```python
from build123d import *

# Parameters (mm, degrees)
BOSS_EXTRUDE1_DEPTH = 35
SKETCH3_W           = 28
SKETCH3_H           = 14
CUT_EXTRUDE1_DEPTH  = 4
FILLET1_R           = 1
SKETCH4_R           = 2
CUT_EXTRUDE2_DEPTH  = 63.072538211


with BuildPart() as part:
    # Sketch2 → Boss-Extrude1 (new body)
    with BuildSketch(Plane.XY):
        Polygon((0, 0), (0, 2), (10, 2), (10, 18), (38, 18), (38, 2), (48, 2), (48, 0), (36, 0), (36, 16), (12, 16), (12, 0), align=None)
    extrude(amount=BOSS_EXTRUDE1_DEPTH)

    # Sketch3 → Cut-Extrude1 (cut)
    with BuildSketch(Plane(origin=(0, 18, 0), x_dir=(1, 0, 0), z_dir=(0, 1, 0))):
        with Locations((24, -28)):
            Rectangle(SKETCH3_W, SKETCH3_H)
    extrude(amount=-CUT_EXTRUDE1_DEPTH, mode=Mode.SUBTRACT)

    # Fillet1
    fillet1_edges = [part.edges().sort_by_distance(p)[0] for p in [
        (0, 2, 17.5),
        (48, 2, 17.5),
        (10, 18, 10.5),
        (38, 18, 10.5),
    ]]
    fillet(fillet1_edges, radius=FILLET1_R)

    # Sketch4 → Cut-Extrude2 (cut, through all)
    with BuildSketch(Plane(origin=(0, 18, 0), x_dir=(1, 0, 0), z_dir=(0, 1, 0))):
        with Locations(Location((24, -8, 0), (0, 0, 270))):
            Circle(SKETCH4_R)
        with Locations(Location((24, -16, 0), (0, 0, 270))):
            Circle(SKETCH4_R)
        with Locations(Location((42.5, -5, 0), (0, 0, 270))):
            Circle(SKETCH4_R)
        with Locations(Location((42.5, -30, 0), (0, 0, 270))):
            Circle(SKETCH4_R)
        with Locations(Location((4.5, -5, 0), (0, 0, 270))):
            Circle(SKETCH4_R)
        with Locations(Location((4.5, -30, 0), (0, 0, 270))):
            Circle(SKETCH4_R)
    extrude(amount=-CUT_EXTRUDE2_DEPTH, mode=Mode.SUBTRACT)


solid = part.part
```
CAD build for the part. Positions are in the model's coordinates, mm. A direction names the side the tool comes from. Coordinates: 2 decimals unless noted, no trailing zeros. Write each loop counter-clockwise with the first axis right and the second up, starting at its lowest first coordinate (ties: lowest second). Pieces come first, ordered by that corner, then holes. Notation, with made-up numbers: (22, 59) -> (39, 59) arc R28 ccw to (39, 77) -> close; hole circle Ø10 at (34, 77.25). An arc over 180 degrees is marked (long way). Use CSV: the item, a comma, the result in double quotes. Start each with the question number.
Item 1: Wall check: probe 1 along X at (y, z) = (0.6, 30); probe 2 along X at (y, z) = (15.25, 3); probe 3 along X at (y, z) = (16.7, 8). Give the ranges that are in metal, low to high.
Item 2: Band-saw the part on D-D, the plane y = 7. Write the cut outline in (x, z).
Item 3: Tool access for faces 1 (the flat face through (48, 0.5, 17.3)), 2 (the flat face through (12, 8, 17)), 3 (the flat face through (38, 10, 17)), 4 (the cylindrical face through (4.588, 1.014, 3.002)), 5 (the flat face through (5, 2, 17)): list every direction of +Z, -Z, +X, -X, +Y, -Y with a clear straight run to the whole face (end or side of a thin tool).
Item 4: Drop flat-ended pins along their axis: P1, Ø1.6, axis at x = 37, z = 27.5, coming from the +Y side; P2, Ø3, axis at x = 26, y = 15, coming from the +Z side; P3, Ø5, axis at y = 4, z = 15.5, coming from the -X side. Give the stop position or say it passes through.
Item 5: Band-saw the part on B-B, the plane y = 14.5. Write the cut outline in (x, z).
Item 6: Two-plate mould, pull along X, no slides. Class faces 6 (the flat face through (0, 0.5, 17.3)), 7 (the flat face through (37.6, 5, 35)), 8 (the flat face through (24.2, 16, 10.4)): +X half, -X half, draft (parallel to the pull), parting line (faces both ways), or undercut.
Item 7: Band-saw the part on C-C, the plane z = 30. Write the cut outline in (x, y), plus the area to 3 significant figures.
Item 8: Band-saw the part on A-A, the plane z = 8. Write the cut outline in (x, y), plus the area to 3 significant figures.
Response values:
1,probe 1,"x = 0 to 2.5, 6.5 to 12, 36 to 40.5, 44.5 to 48"
1,probe 2,"x = 10 to 12, 36 to 38"
1,probe 3,"x = 10 to 22, 26 to 38"
2,outline,"(10, 0) -> (12, 0) -> (12, 35) -> (10, 35) -> close; (36, 0) -> (38, 0) -> (38, 35) -> (36, 35) -> close"
3,face 1,"+Z, -Z, +X, +Y, -Y"
3,face 2,"+Z, -Z, -Y"
3,face 3,"+Z, -Z, +X, +Y"
3,face 4,"+Y, -Y"
3,face 5,"+Z, -Z, -X, +Y"
4,P1,"stops at y = 14"
4,P2,"stops at z = 21"
4,P3,"stops at x = 0.13"
5,outline,"(10, 0) -> (12, 0) -> (12, 21) -> (10, 21) -> close; (36, 0) -> (38, 0) -> (38, 21) -> (36, 21) -> close"
6,face 6,"-X half"
6,face 7,"draft"
6,face 8,"undercut"
7,outline,"(0, 0) -> (2.5, 0) -> (2.5, 2) -> (1, 2) arc R1 ccw to (0, 1) -> close; (6.5, 0) -> (12, 0) -> (12, 14) -> (10, 14) -> (10, 2) -> (6.5, 2) -> close; (36, 0) -> (40.5, 0) -> (40.5, 2) -> (38, 2) -> (38, 14) -> (36, 14) -> close; (44.5, 0) -> (48, 0) -> (48, 1) arc R1 ccw to (47, 2) -> (44.5, 2) -> close"
7,area,"79.6 mm2"
8,outline,"(0, 0) -> (12, 0) -> (12, 16) -> (22, 16) -> (22, 18) -> (11, 18) arc R1 ccw to (10, 17) -> (10, 2) -> (1, 2) arc R1 ccw to (0, 1) -> close; (26, 16) -> (36, 16) -> (36, 0) -> (48, 0) -> (48, 1) arc R1 ccw to (47, 2) -> (38, 2) -> (38, 17) arc R1 ccw to (37, 18) -> (26, 18) -> close"
8,area,"151 mm2"
